The listing builds one solid part. Answer for the finished solid, in the listing's coordinates (mm). A direction names the side the tool comes from. Give positions to 0.01 mm unless a question says otherwise; leave off trailing zeros. Order: outer loops, then holes, each group sorted by start corner. A loop starts at its lowest first (then second) coordinate and runs counter-clockwise, first axis right, second up. Notation, with made-up numbers: (21.25, 60.25) - (28.25, 60.25) arc R12 cw to (28.25, 82.25) - close; hole circle Ø11 at (80.25, -30.5). An arc over 180 degrees is marked (long way). Answer as a JSON object with one key per item and string values. Group by question number.
Q1. Consider line 1 (Z direction, x = -4.2, y = 0); line 2 (X direction, y = -1, z = 57.5); line 3 (Y direction, x = 4.15, z = 5). Determine where each line is inside the solid, lowest interval first.
Q2. The mould has two halves that part along Y. Classify faces 3 (the face through (4.5, 0, 42)), 4 (the face through (-3.75, 0, 42)), 5 (the face through (0, -4.5, 42)): released by +Y, released by -Y, zero draft, split by the parting line, or undercut.
Q3. A cutting plane is placed at B-B, the plane z = 18. Give the vertices of the cut face in (x, y).
Q4. A cutting plane is placed at A-A, the plane x = -3. Give the vertices of the cut face in (y, z), and give its area (4 significant figures).
Q5. A cutting plane is placed at D-D, the plane z = 5. Give the vertices of the cut face in (x, y), and give its area (4 significant figures).
Q6. Given pin 1 (3 mm diameter, centred on y = 0, z = 5, fed in from +X), flat-ended and moving along its own axis, determine where the tip first touches the part or whether it passes through.
Q7. For faces 1 (the face through (0, 3.75, 42)), 2 (the face through (-4.13, -1.08, 26.18)), determine the directions among +Z, -Z, +X, -X, +Y, -Y from which every point of the face is accessible in a straight line to the end or side of a thin tool.
Autodesk Inventor part; units mm, degrees
ref_plane "YZ Plane" through (0, 0, 0) normal (1, 0, 0) x (0, 1, 0)
ref_plane "XZ Plane" through (0, 0, 0) normal (0, 1, 0) x (-1, 0, 0)
ref_plane "XY Plane" through (0, 0, 0) normal (0, 0, 1) x (1, 0, 0)
sketch "スケッチ1" plane through (0, 0, 0) normal (0, 0, 1) x (1, 0, 0)
  line L0 (4.5, -4.5) -> (-4.5, -4.5)
  line L1 (-4.5, -4.5) -> (-4.5, 4.5)
  line L2 (-4.5, 4.5) -> (4.5, 4.5)
  line L3 (4.5, 4.5) -> (4.5, -4.5)
  line L4 (4.5, -4.5) -> (-4.5, 4.5) construction
  line L5 (-4.5, -4.5) -> (4.5, 4.5) construction
  line L6 (3.75, -3.75) -> (-3.75, -3.75)
  line L7 (-3.75, -3.75) -> (-3.75, 3.75)
  line L8 (-3.75, 3.75) -> (3.75, 3.75)
  line L9 (3.75, 3.75) -> (3.75, -3.75)
  line L10 (3.75, -3.75) -> (-3.75, 3.75) construction
  line L11 (-3.75, -3.75) -> (3.75, 3.75) construction
  point P0 (0, 0)
  dimension "d0" = 9
  dimension "d1" = 9
  dimension "d2" = 7.5
  dimension "d3" = 7.5
extrude "押し出し1" add sketch "スケッチ1" along normal blind 90
sketch "スケッチ2" plane through (4.5, -4.5, 0) normal (1, 0, 0) x (0, 0, -1)
  line L0 (0, 0) -> (-90, 0)
  line L1 (0, 0) -> (0, 9)
  point P0 (0, 4.5)
  point P1 (-5, 4.5)
  point P2 (-25, 4.5)
  point P3 (-45, 4.5)
  dimension "d6" = 4.5
  dimension "d7" = 5
  dimension "d8" = 20
  dimension "d9" = 20
hole "穴1" at (4.5, 0, 5) at (4.5, 0, 25) at (4.5, 0, 45) direction (-1, 0, 0) diameter 3.2 end through all
sketch "スケッチ3" plane through (0, 0, 90) normal (0, 0, 1) x (1, 0, 0)
  line L0 (4.5, -4.5) -> (-4.5, -4.5)
  line L1 (-4.5, -4.5) -> (-4.5, 4.5)
  line L2 (-4.5, 4.5) -> (4.5, 4.5)
  line L3 (4.5, 4.5) -> (4.5, -4.5)
  line L4 (4.5, -4.5) -> (-4.5, 4.5) construction
  line L5 (-4.5, -4.5) -> (4.5, 4.5) construction
  point P0 (0, 0)
extrude "押し出し2" cut sketch "スケッチ3" against normal blind 5
properties part number "squareEx1"
Reply:
{
 "1": {"line 1": "z = 0 to 3.4, 6.6 to 23.4, 26.6 to 43.4, 46.6 to 85", "line 2": "x = -4.5 to -3.75, 3.75 to 4.5", "line 3": "y = -4.5 to -1.6, 1.6 to 4.5"},
 "2": {"face 3": "zero draft", "face 4": "undercut", "face 5": "released by -Y"},
 "3": {"outline": "(-4.5, -4.5) - (4.5, -4.5) - (4.5, 4.5) - (-4.5, 4.5) - close; hole (-3.75, -3.75) - (3.75, -3.75) - (3.75, 3.75) - (-3.75, 3.75) - close"},
 "4": {"outline": "(-4.5, 0) - (-3.75, 0) - (-3.75, 85) - (-4.5, 85) - close; (3.75, 0) - (4.5, 0) - (4.5, 85) - (3.75, 85) - close", "area": "127.5 mm^2"},
 "5": {"outline": "(-4.5, -4.5) - (4.5, -4.5) - (4.5, -1.6) - (3.75, -1.6) - (3.75, -3.75) - (-3.75, -3.75) - (-3.75, -1.6) - (-4.5, -1.6) - close; (-4.5, 1.6) - (-3.75, 1.6) - (-3.75, 3.75) - (3.75, 3.75) - (3.75, 1.6) - (4.5, 1.6) - (4.5, 4.5) - (-4.5, 4.5) - close", "area": "19.95 mm^2"},
 "6": {"pin 1": "passes through"},
 "7": {"face 1": "+Z, -Z", "face 2": "+X, -X"}
}
